The figure shows three views and two pictorial views of one solid part (mm, origin at its lowest corner). Answer the questions. Give positions to 0.01 mm unless a question says otherwise; leave off trailing zeros. Loops run counter-clockwise (first coordinate to the right, second up) from the corner with the lowest first, then second, coordinate; pieces in that order, holes last. Notation, with made-up numbers: M -28.75,23.25 L 1.25,23.25 A11 cw 1.25,44.25 Z; hole C 68.5,6.25 d4. An arc over 180 degrees is marked long. Answer as a JSON object with one key per item and string values. Group by question number.
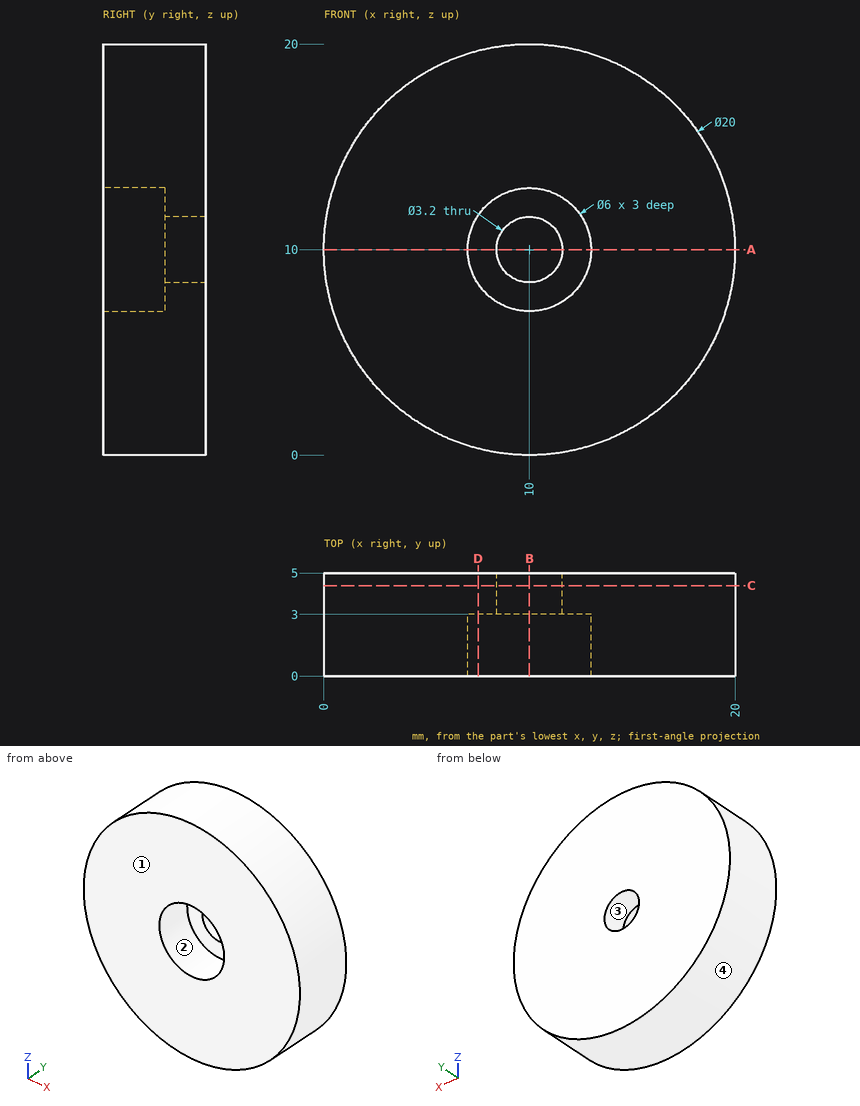
Item 1: Given pin 1 Ø5 at (x, z) = (10, 7) entering from -Y; pin 2 Ø1.8 at (x, z) = (9, 11.5) entering from -Y; pin 3 Ø3 at (y, z) = (2, 14.5) entering from +X; pin 4 Ø1.9 at (x, z) = (10, 10) entering from +Y, each flat-ended and moving along its own axis, determine where each tip first touches the part or whether it passes through.
Item 2: A cutting plane is placed at D-D (x = 7.5). Determine the outline of the cut face in (y, z).
Item 3: A cutting plane is placed at B-B (x = 10). Determine the outline of the cut face in (y, z), and give its area (3 significant figures).
Item 4: A cutting plane is placed at A-A (z = 10). Determine the outline of the cut face in (x, y).
Item 5: A cutting plane is placed at C-C (y = 4.4). Determine the outline of the cut face in (x, z), and give its area (3 significant figures).
Item 6: Find the intervals of material crossed by probe 1 along X at (y, z) = (0.65, 10); probe 2 along X at (y, z) = (3.4, 10); probe 3 along Y at (x, z) = (7.25, 10.25), in increasing order. Write a range as [from, to].
Item 7: For a pull along X with two mould halves and no side action, classify the marked faces 1, 2, 3 and 4 as pulls with the +X half, pulls with the -X half, needs draft (parallel to the pull), parting line crosses it, or undercut.
The answers:
{
 "1": {"pin 1": "stops at y = 0", "pin 2": "stops at y = 3", "pin 3": "stops at x = 19.54", "pin 4": "passes through"},
 "2": {"outline": "M 0,0.32 L 5,0.32 L 5,19.68 L 0,19.68 L 0,11.66 L 3,11.66 L 3,8.34 L 0,8.34 Z"},
 "3": {"outline": "M 0,0 L 5,0 L 5,8.4 L 3,8.4 L 3,7 L 0,7 Z; M 0,13 L 3,13 L 3,11.6 L 5,11.6 L 5,20 L 0,20 Z", "area": "75.6 mm^2"},
 "4": {"outline": "M 0,0 L 7,0 L 7,3 L 8.4,3 L 8.4,5 L 0,5 Z; M 11.6,3 L 13,3 L 13,0 L 20,0 L 20,5 L 11.6,5 Z"},
 "5": {"outline": "C 10,10 d20; hole C 10,10 d3.2", "area": "306 mm^2"},
 "6": {"probe 1": "x = [0, 7], [13, 20]", "probe 2": "x = [0, 8.4], [11.6, 20]", "probe 3": "y = [3, 5]"},
 "7": {"face 1": "needs draft", "face 2": "undercut", "face 3": "undercut", "face 4": "parting line crosses it"}
}
